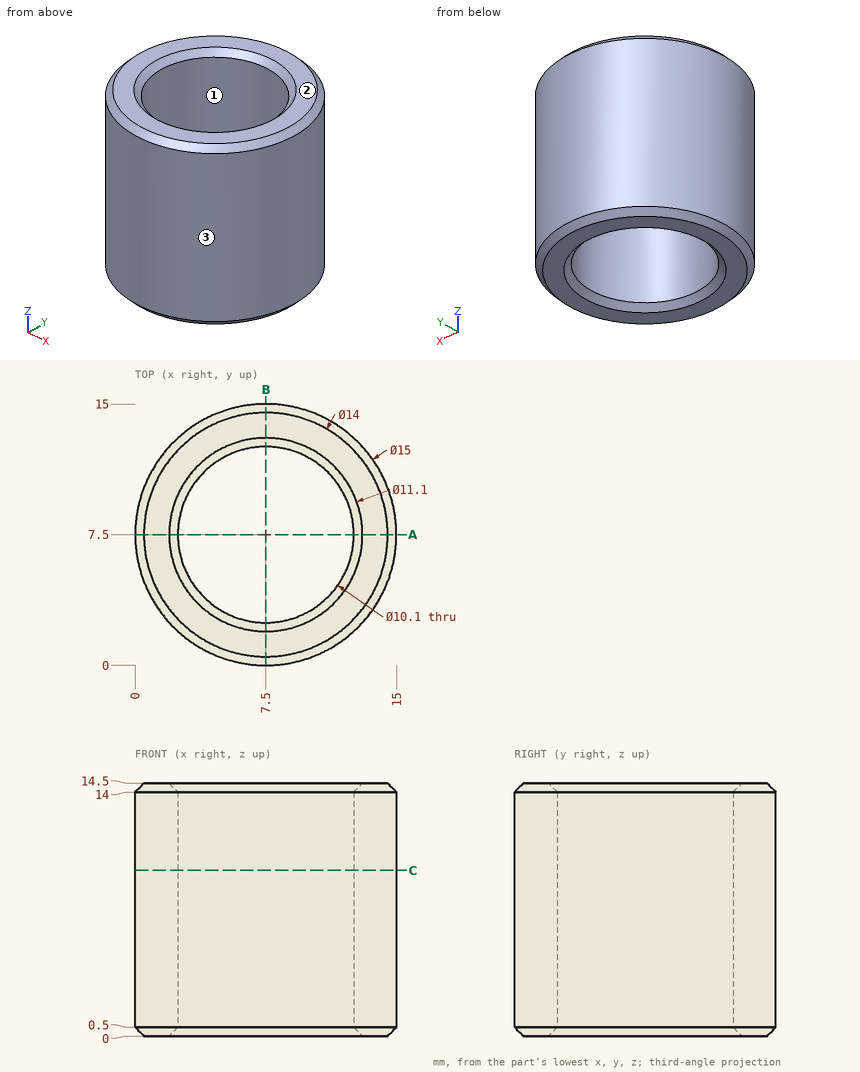
Study the drawing (mm; zero at the part's minimum x, y, z) and answer. Coordinates: 2 decimals unless noted, no trailing zeros. Write each loop counter-clockwise with the first axis right and the second up, starting at its lowest first coordinate (ties: lowest second). Pieces come first, ordered by that corner, then holes. Notation, with made-up numbers: (38, 80) - (67, 80) arc R26 ccw to (67, 94) - close; hole circle Ø10 at (88, 12.25). An arc over 180 degrees is marked (long way). One line per question, with ' | ' between items.
1) The mould has two halves that part along Y. Classify the marked faces 1, 2 and 3: +Y half, -Y half, draft (parallel to the pull), parting line (faces both ways), or undercut.
Checks:
face 1: undercut | face 2: draft | face 3: parting line
2) Find section A-A, the plane y = 7.5. Determine the outline of the cut face in (x, z), and give its area (4 significant figures).
Checks:
outline: (0, 0.5) - (0.5, 0) - (1.95, 0) - (2.45, 0.5) - (2.45, 14) - (1.95, 14.5) - (0.5, 14.5) - (0, 14) - close; (12.55, 0.5) - (13.05, 0) - (14.5, 0) - (15, 0.5) - (15, 14) - (14.5, 14.5) - (13.05, 14.5) - (12.55, 14) - close | area: 70.05 mm2
3) Consider probe 1 along Y at (x, z) = (7.5, 10.5); probe 2 along Y at (x, z) = (3.75, 11.75); probe 3 along X at (y, z) = (5, 9.75). Determine where each line is inside the solid, lowest interval first. Write a range as [from, to].
Checks:
probe 1: [0, 2.45], [12.55, 15] | probe 2: [1, 4.12], [10.88, 14] | probe 3: [0.43, 3.11], [11.89, 14.57]
4) Flat-ended cylindrical pins translate along their axes: P1, Ø4, axis at y = 2.5, z = 6, coming from the +X side; P2, Ø1.5, axis at y = 4.5, z = 7, coming from the -X side; P3, Ø1.5, axis at x = 12.5, z = 3, coming from the +Y side. Find the tip coordinate at first contact, or state that the pin passes through.
Checks:
P1: x = 14.37 | P2: x = 0.35 | P3: y = 13.68
5) Find section C-C, the plane z = 9.5. Determine the outline of the cut face in (x, y).
Checks:
outline: circle Ø15 at (7.5, 7.5); hole circle Ø10.1 at (7.5, 7.5)
